from build123d import *

# Parameters (mm, degrees)
SKETCH1_R           = 2.8
BOSS_EXTRUDE1_DEPTH = 1.5
FILLET1_R           = 1
SKETCH2_R           = 1.5
BOSS_EXTRUDE2_DEPTH = 10


with BuildPart() as part:
    # Sketch1 → Boss-Extrude1 (new body)
    with BuildSketch(Plane(origin=(0, 0, 0), x_dir=(1, 0, 0), z_dir=(0, 1, 0))):
        with Locations(Location((0, 0, 0), (0, 0, 270))):
            Circle(SKETCH1_R)
    extrude(amount=BOSS_EXTRUDE1_DEPTH)

    # Fillet1
    fillet1_edges = [part.edges().sort_by_distance(p)[0] for p in [
        (0, 1.5, -2.8),
    ]]
    fillet(fillet1_edges, radius=FILLET1_R)

    # Sketch2 → Boss-Extrude2 (add)
    with BuildSketch(Plane.XZ):
        with Locations(Location((0, 0, 0), (0, 0, 270))):
            Circle(SKETCH2_R)
    extrude(amount=BOSS_EXTRUDE2_DEPTH)


solid = part.part
Build history of the part. All positions in model axes, mm. A direction names the side the tool comes from. Round coordinates to 2 decimals unless told otherwise and drop trailing zeros. Loops run counter-clockwise (first coordinate to the right, second up) from the corner with the lowest first, then second, coordinate; pieces in that order, holes last. Notation, with made-up numbers: (-34, 76.5) -> (15, 76.5) arc R13 ccw to (15, 82.5) -> close; hole circle Ø1 at (46.5, 79). An arc over 180 degrees is marked (long way). One line per item, written item: value. Start each with the question number.
Q1. Cut at B-B on x = 0. List the corners of the cut face in (y, z).
Q2. Cut at C-C on y = -2. List the corners of the cut face in (x, z), plus the area to 3 significant figures.
Q3. 3-axis set-ups, long thin cutter, end or side, ignore diameter. For faces 1 (the face through (0, -10, 0)), 2 (the face through (0.45, -4.93, -1.43)): which of +Z, -Z, +X, -X, +Y, -Y reach the whole face in a straight line?
Q4. Probe line 1 along Y through (x, z) = (1.15, -1.4); line 2 along Z through (x, y) = (0.05, -3); line 3 along Z through (x, y) = (2.1, 0.75). List the from-to ranges inside material, lowest first.
Q5. Drop flat-ended pins along their axis: pin 1 Ø1 at (x, y) = (0, -2) entering from +Z; pin 2 Ø1.5 at (y, z) = (0, 1.5) entering from -X; pin 3 Ø1.5 at (y, z) = (-1.5, -0.5) entering from -X; pin 4 Ø2 at (x, z) = (-1.5, 1) entering from -Y. Give the stop position or say it passes through.
Q6. Cut at A-A on z = 0. List the corners of the cut face in (x, y).
Computed:
1. outline: (-10, -1.5) -> (0, -1.5) -> (0, -2.8) -> (0.5, -2.8) arc R1 ccw to (1.5, -1.8) -> (1.5, 1.8) arc R1 ccw to (0.5, 2.8) -> (0, 2.8) -> (0, 1.5) -> (-10, 1.5) -> close
2. outline: circle Ø3 at (0, 0)
2. area: 7.07 mm²
3. face 1: +Z, -Z, +X, -X, -Y
3. face 2: -Y
4. line 1: 0 to 1.5
4. line 2: -1.5 to 1.5
4. line 3: -1.8 to 1.8
5. pin 1: z = 1.5
5. pin 2: x = -2.7
5. pin 3: x = -1.5
5. pin 4: y = -10
6. outline: (-2.8, 0) -> (-1.5, 0) -> (-1.5, -10) -> (1.5, -10) -> (1.5, 0) -> (2.8, 0) -> (2.8, 0.5) arc R1 ccw to (1.8, 1.5) -> (-1.8, 1.5) arc R1 ccw to (-2.8, 0.5) -> close
